Can you work these out from the model? Positions are in its coordinate system, mm. Face numbers are marked on the shaded views. A direction names the side the tool comes from. Round coordinates to 2 decimals unless told otherwise and drop trailing zeros. Order: outer loops, then holes, each group sorted by start corner. A loop starts at its lowest first (then second) coordinate and runs counter-clockwise, first axis right, second up.
from build123d import *

# Parameters (mm, degrees)
REVOLVE_THIN1_ANGLE = 285


with BuildPart() as part:
    # Sketch1 → Revolve-Thin1 (revolve)
    with BuildSketch(Plane.XY):
        with BuildLine():
            Line((-27.538484773, 20.124551934), (-27.538484773, 15.403929488))
            Line((-27.538484773, 15.403929488), (-36.227206247, 15.403929488))
            Line((-36.227206247, 15.403929488), (-36.227206247, -4))
            Line((-36.227206247, -4), (-6.746755937, -4))
            Line((-6.746755937, -4), (-6.746755937, 38.091146669))
            Line((-6.746755937, 38.091146669), (-22.039284373, 38.091146669))
            ThreePointArc((-22.039284373, 38.091146669), (-20.717051221, 33.270500036), (-23.203151183, 28.933883676))
            ThreePointArc((-23.203151183, 28.933883676), (-26.395944189, 25.033712837), (-27.538484773, 20.124551934))
        make_face()
        with BuildLine():
            Line((-23.538484773, 20.124551934), (-23.538484773, 11.403929488))
            Line((-23.538484773, 11.403929488), (-32.227206247, 11.403929488))
            Line((-32.227206247, 11.403929488), (-32.227206247, 0))
            Line((-32.227206247, 0), (-10.746755937, 0))
            Line((-10.746755937, 0), (-10.746755937, 34.091146669))
            Line((-10.746755937, 34.091146669), (-16.665109009, 34.091146669))
            ThreePointArc((-16.665109009, 34.091146669), (-17.745052772, 29.450945899), (-20.762920969, 25.764455257))
            ThreePointArc((-20.762920969, 25.764455257), (-22.807008354, 23.267491001), (-23.538484773, 20.124551934))
        make_face(mode=Mode.SUBTRACT)
    revolve(axis=Axis((0, 0, 0), (0, 1, 0)), revolution_arc=REVOLVE_THIN1_ANGLE)


solid = part.part
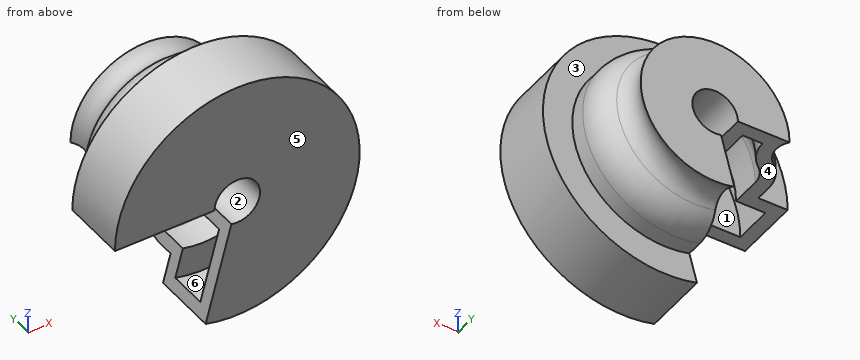
(1) I want a section at C-C, the plane y = 1. List the corners of the cut face in (x, z) for me.
(2) I want a section at B-B, the plane y = 17.5. List the corners of the cut face in (x, z) for me.
(3) I want a section at A-A, the plane x = 0. Give the number of separate pieces and of enclosed holes in the cut face, plus the area to 3 significant figures.
(4) On a 3-axis mill with a long thin cutter (end or side, diameter ignored), from which of +Z, -Z, +X, -X, +Y, -Y can I reach the whole of each face in a straight line? I mean the marked faces 4, 5 and 6. Say none if no direction works.
(5) Please list where these lines run through material, in increasing order: probe 1 along Z at (x, y) = (0, 4); probe 2 along Z at (x, y) = (0, 14.5); probe 3 along Y at (x, z) = (29.5, -6).
(6) I want a section at D-D, the plane x = 29.5. List the corners of the cut face in (y, z) for me, plus the area to 3 significant figures.
(7) If we mould it in two halves opening along Y, with no side actions, what happens to the marked faces 1, 2 and 3? For each: pulls with the +Y half, pulls with the -Y half, needs draft (parallel to the pull), parting line crosses it, or undercut.
(8) I'm going to push flat-ended pins straight in: pin 1 Ø12 at (x, y) = (22.5, 11.5) entering from +Z; pin 2 Ø10 at (x, y) = (-4, 12.5) entering from +Z; pin 3 Ø1.5 at (x, y) = (19, 2.5) entering from +Z; pin 4 Ø10 at (x, z) = (4, 0.5) entering from -Y. Where does each tip first touch, or does it pass through?
Ans:
1. outline: (-36.23, 0) - (-32.23, 0) arc R32.23 cw (long way) to (-8.34, -31.13) - (-9.38, -34.99) arc R36.23 ccw (long way) to start; (-10.75, 0) - (-6.75, 0) arc R6.75 cw (long way) to (-1.75, -6.52) - (-2.78, -10.38) arc R10.75 ccw (long way) to start
2. outline: (-27.54, 0) - (-23.54, 0) arc R23.54 cw (long way) to (-6.09, -22.74) - (-7.13, -26.6) arc R27.54 ccw (long way) to start; (-10.75, 0) - (-6.75, 0) arc R6.75 cw (long way) to (-1.75, -6.52) - (-2.78, -10.38) arc R10.75 ccw (long way) to start
3. separate pieces: 2
3. enclosed holes: 2
3. area: 983 mm2
4. face 4: -X, +Y, -Y
4. face 5: +Z, -Z, +X, -X, -Y
4. face 6: none
5. probe 1: z = -36.23 to -32.23, -10.75 to -6.75, 6.75 to 10.75, 32.23 to 36.23
5. probe 2: z = -36.23 to -23.54, -10.75 to -6.75, 6.75 to 10.75, 23.54 to 36.23
5. probe 3: y = -4 to 0, 11.4 to 15.4
6. outline: (-4, -21.03) - (15.4, -21.03) - (15.4, 21.03) - (-4, 21.03) - close; hole (0, -12.97) - (11.4, -12.97) - (11.4, 12.97) - (0, 12.97) - close
6. area: 520 mm2
7. face 1: undercut
7. face 2: needs draft
7. face 3: pulls with the +Y half
8. pin 1: stops at z = 32.25
8. pin 2: stops at z = 36.23
8. pin 3: stops at z = 31.29
8. pin 4: stops at y = -4
